The model under review builds one solid part; all positions refer to its coordinate system, in mm. Give positions to 0.01 mm unless a question says otherwise; leave off trailing zeros. Order: outer loops, then holes, each group sorted by start corner. A loop starts at its lowest first (then second) coordinate and runs counter-clockwise, first axis right, second up. Notation, with made-up numbers: (56.5, 44) - (71.5, 44) arc R29 ccw to (71.5, 78) - close; hole circle Ø3 at (-38.75, 86.5). An arc over 180 degrees is marked (long way). Use CSV: the item, a comma, the result in double quotes. Start each with the question number.
1. Take a section at D-D, the plane y = -4. State the section outline as (x, z) points.
2. Take a section at A-A, the plane y = 0. State the section outline as (x, z) points.
3. To check wall thickness, follow line 1 (X direction, y = -2.25, z = 0.15); line 2 (X direction, y = 4, z = 0.15); line 3 (Y direction, x = 1.75, z = 0.05). State the ranges of each line that lie inside material, in increasing order. Write a range as [from, to].
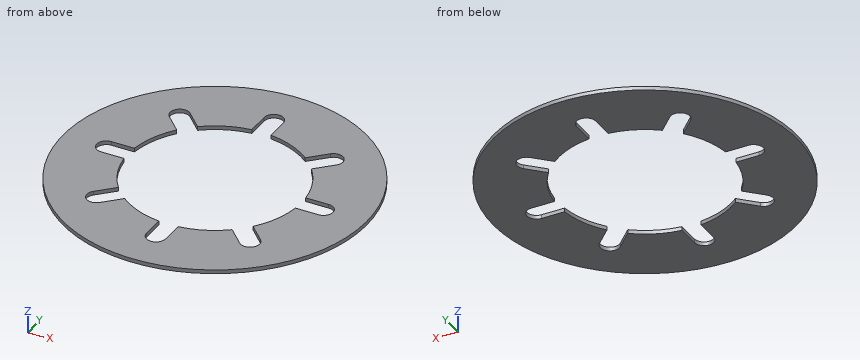
```python
from build123d import *

# Parameters (mm, degrees)
F0_R     = 7.9
F1_DEPTH = 0.2


with BuildPart() as f1:
    # F0 (on Top) → F1 (new body)
    with BuildSketch(Plane.XY):
        Circle(F0_R)
        with BuildLine():
            ThreePointArc((-2.808724, 3.515831), (-1.722075, 4.157458), (-0.5, 4.472136))
            Line((-0.5, 4.472136), (-0.5, 5.672136))
            ThreePointArc((-0.5, 5.672136), (0, 6.172136), (0.5, 5.672136))
            Line((0.5, 5.672136), (0.5, 4.472136))
            ThreePointArc((0.5, 4.472136), (1.722075, 4.157458), (2.808724, 3.515831))
            Line((2.808724, 3.515831), (3.657252, 4.364359))
            ThreePointArc((3.657252, 4.364359), (4.364359, 4.364359), (4.364359, 3.657252))
            Line((4.364359, 3.657252), (3.515831, 2.808724))
            ThreePointArc((3.515831, 2.808724), (4.157458, 1.722075), (4.472136, 0.5))
            Line((4.472136, 0.5), (5.672136, 0.5))
            ThreePointArc((5.672136, 0.5), (6.172136, 0), (5.672136, -0.5))
            Line((5.672136, -0.5), (4.472136, -0.5))
            ThreePointArc((4.472136, -0.5), (4.157458, -1.722075), (3.515831, -2.808724))
            Line((3.515831, -2.808724), (4.364359, -3.657252))
            ThreePointArc((4.364359, -3.657252), (4.364359, -4.364359), (3.657252, -4.364359))
            Line((3.657252, -4.364359), (2.808724, -3.515831))
            ThreePointArc((2.808724, -3.515831), (1.722075, -4.157458), (0.5, -4.472136))
            Line((0.5, -4.472136), (0.5, -5.672136))
            ThreePointArc((0.5, -5.672136), (0, -6.172136), (-0.5, -5.672136))
            Line((-0.5, -5.672136), (-0.5, -4.472136))
            ThreePointArc((-0.5, -4.472136), (-1.722075, -4.157458), (-2.808724, -3.515831))
            Line((-2.808724, -3.515831), (-3.657252, -4.364359))
            ThreePointArc((-3.657252, -4.364359), (-4.364359, -4.364359), (-4.364359, -3.657252))
            Line((-4.364359, -3.657252), (-3.515831, -2.808724))
            ThreePointArc((-3.515831, -2.808724), (-4.157458, -1.722075), (-4.472136, -0.5))
            Line((-4.472136, -0.5), (-5.672136, -0.5))
            ThreePointArc((-5.672136, -0.5), (-6.172136, 0), (-5.672136, 0.5))
            Line((-5.672136, 0.5), (-4.472136, 0.5))
            ThreePointArc((-4.472136, 0.5), (-4.157458, 1.722075), (-3.515831, 2.808724))
            Line((-3.515831, 2.808724), (-4.364359, 3.657252))
            ThreePointArc((-4.364359, 3.657252), (-4.364359, 4.364359), (-3.657252, 4.364359))
            Line((-3.657252, 4.364359), (-2.808724, 3.515831))
        make_face(mode=Mode.SUBTRACT)
    extrude(amount=F1_DEPTH)


solid = f1.part
```
Determined:
1,outline,"(-6.81, 0) - (-4.51, 0) - (-4.51, 0.2) - (-6.81, 0.2) - close; (-3.29, 0) - (-2.06, 0) - (-2.06, 0.2) - (-3.29, 0.2) - close; (2.06, 0) - (3.29, 0) - (3.29, 0.2) - (2.06, 0.2) - close; (4.51, 0) - (6.81, 0) - (6.81, 0.2) - (4.51, 0.2) - close"
2,outline,"(-7.9, 0) - (-6.17, 0) - (-6.17, 0.2) - (-7.9, 0.2) - close; (6.17, 0) - (7.9, 0) - (7.9, 0.2) - (6.17, 0.2) - close"
3,line 1,"x = [-7.57, -3.9], [3.9, 7.57]"
3,line 2,"x = [-6.81, -4.51], [-3.29, -2.06], [2.06, 3.29], [4.51, 6.81]"
3,line 3,"y = [-7.7, -4.15], [4.15, 7.7]"
